Input: part model. Units: mm. Frame: model coordinates. Give positions to 0.01 mm unless a question says otherwise; leave off trailing zeros. Use CSV: the item, a comma, the result in double quotes. Start each with the question number.
Q1. Material intervals for line 1 along Y through (x, z) = (51, 8.5); line 2 along X through (y, z) = (-22, -9); line 3 along X through (y, z) = (-117.5, 9), sorted ascending.
Q2. Pull-direction query (Y, two-part tool) for faces 1 (the flat face through (118.296, 15.61, 0.627)), 2 (the flat face through (0, 0, 1)), 3 (the cylindrical face through (128.32, -125.56, -5.77)); classes: released by +Y, released by -Y, zero draft, split by the parting line, or undercut.
Q3. Pin query (flat end, axial travel): pin 1 (4 mm diameter, centred on y = -250, z = 11, fed in from +X); pin 2 (8 mm diameter, centred on x = 57, z = -7.5, fed in from +Y); pin 3 (10 mm diameter, centred on y = -74, z = -13.5, fed in from -X); pin 4 (10 mm diameter, centred on x = 159, z = 0, fed in from -Y). Return the tip coordinate at first contact, or that it passes through.
from build123d import *

# Parameters (mm, degrees)
CROQUIS8_R              = 12.5
SALIENTE_EXTRUIR1_REACH = 326.791
CROQUIS11_R             = 12.5


with BuildPart() as part:
    # Barrer2: sweep along a path in Croquis7
    with BuildLine() as barrer2_path:  # in the path sketch's own coordinates; laid on its plane below (add() does not lay a ready-made edge on the line's plane)
        add(Edge.make_bspline(
            [(0, 0), (40.063845147, 12.936685998), (79.927373916, -21.140368078), (118.219501425, 15.689998663)],
            knots=[0, 0, 0, 0, 1, 1, 1, 1], degree=3))
    # Croquis8 → Barrer2 (sweep)
    with BuildSketch(Plane(origin=(0, 0, 0), x_dir=(0, 0, -1), z_dir=(0.9516192950583919, 0.30727954255460815, 0))):
        Circle(CROQUIS8_R)
    sweep(path=Plane.XY * barrer2_path.line)

    # Croquis11 → Saliente-Extruir1 (add, up to next)
    with BuildSketch(Plane(origin=(163.655125908, -253.290566887, 0), x_dir=(0.9381132106931296, 0.34632875122205475, 0), z_dir=(-0.34632875122205475, 0.9381132106931296, 0)), mode=Mode.PRIVATE) as saliente_extruir1_sk1:
        with Locations(Location((0, 0, 0), (0, 0, 90))):
            Circle(CROQUIS11_R)
    saliente_extruir1_tool1 = extrude(saliente_extruir1_sk1.sketch, amount=SALIENTE_EXTRUIR1_REACH, mode=Mode.PRIVATE) - part.part
    add(saliente_extruir1_tool1.solids().sort_by_distance((163.655126, -253.290567, 0))[0])

    # Croquis12 → Revolución3 (revolve)
    with BuildSketch(Plane.XY):
        Polygon((163.655125908, -253.290566887), (175.381541042, -248.961457497), (198.146766592, -283.195862788), (177.508275957, -290.815095315), align=None)
    revolve(axis=Axis((177.508275957, -290.815095315, 0), (-0.34632875122205564, 0.9381132106931294, 0)))


solid = part.part
A:
1,line 1,"-9.21 to 9.31"
1,line 2,"69.02 to 87.52"
1,line 3,"104.28 to 122.77"
2,face 1,"released by +Y"
2,face 2,"released by -Y"
2,face 3,"undercut"
3,pin 1,"x = 172.03"
3,pin 2,"y = 11.44"
3,pin 3,"x = 87.37"
3,pin 4,"y = -298.43"
